Check sheet for the modelled part. Datum: model origin and axes. Units: mm. Face numbers are marked on the shaded views. A direction names the side the tool comes from. Give positions to 0.01 mm unless a question says otherwise; leave off trailing zeros. Loops run counter-clockwise (first coordinate to the right, second up) from the corner with the lowest first, then second, coordinate; pieces in that order, holes last. Notation, with made-up numbers: (41, 18.25) - (82, 18.25) arc R21 ccw to (82, 23.25) - close; hole circle Ø4 at (18.25, 0.25). An arc over 180 degrees is marked (long way). Use CSV: the item, a comma, the result in double quotes.
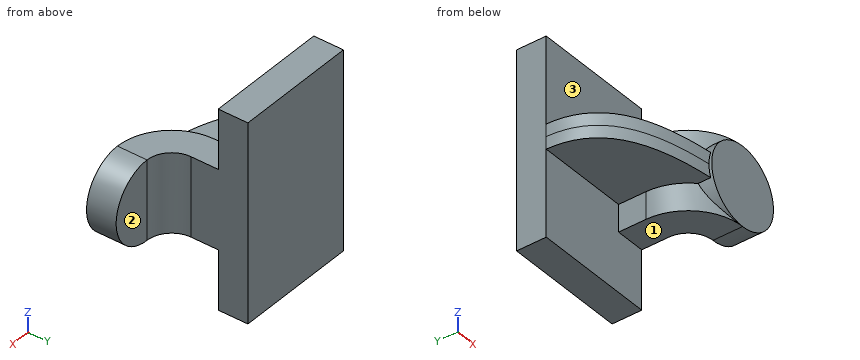
from build123d import *

# Parameters (mm, degrees)
F1_DEPTH = 63.5
F2_DEPTH = 25.4
F3_DEPTH = 7.9375
F0_W     = 25.4
F0_H     = 19.0500014678


with BuildPart() as f1:
    # F0 (on Top) → F1 (new body, symmetric)
    with BuildSketch(Plane.XY):
        Polygon((39.2749942839, 9.525), (-39.2749942839, 9.525), (-39.2749942839, -9.525), (20.2249928161, -9.525), (39.2749942839, -9.525), align=None)
    extrude(amount=F1_DEPTH, both=True)

    # F0 (on Top) → F2 (join, symmetric)
    with BuildSketch(Plane.XY):
        with BuildLine():
            Line((39.2749942839, -27.0002), (39.2749942839, -9.525))
            Line((39.2749942839, -9.525), (20.2249928161, -9.525))
            Line((20.2249928161, -9.525), (20.2249928161, -27.0002))
            ThreePointArc((20.2249928161, -27.0002), (29.3367398508, -50.5253274831), (51.9175683258, -61.7752938165))
            add(Edge.make_bspline(
                [(51.9175683258, -61.7752938165), (52.9952696281, -61.8278519925), (54.0729461799, -61.8776803226), (55.1499942839, -61.9252014678)],
                knots=[105.4761775762, 105.4761775762, 105.4761775762, 105.4761775762, 107.990090193, 107.990090193, 107.990090193, 107.990090193], degree=3))
            Line((55.1499942839, -61.9252014678), (55.1499942839, -42.8752))
            ThreePointArc((55.1499942839, -42.8752), (43.9246741326, -38.2255201513), (39.2749942839, -27.0002))
        make_face()
    extrude(amount=F2_DEPTH, both=True)

    # F0 (on Top) → F3 (join, symmetric)
    with BuildSketch(Plane.XY):
        with BuildLine():
            Line((20.2249928161, -9.525), (-39.2749942839, -9.525))
            add(Edge.make_bspline(
                [(-39.2749942839, -9.525), (-38.560182874, -52.5593411678), (6.7004779731, -59.5701115574), (51.9175683258, -61.7752938165)],
                knots=[0, 0, 0, 0, 105.4761775762, 105.4761775762, 105.4761775762, 105.4761775762], degree=3))
            ThreePointArc((51.9175683258, -61.7752938165), (29.3367398508, -50.5253274831), (20.2249928161, -27.0002))
            Line((20.2249928161, -27.0002), (20.2249928161, -9.525))
        make_face()
    extrude(amount=F3_DEPTH, both=True)

    # F0 (on Top) → F4 (revolve)
    with BuildSketch(Plane.XY):
        with Locations((67.8499942839, -52.4002007339)):
            Rectangle(F0_W, F0_H)
    revolve(axis=Axis((55.1499942839, -52.3875, 0), (0, -1, 0)))


solid = f1.part
1. Sectioned sample at D-D, the plane z = -45.5. Record the boundary of the cut face in (x, y) (3 decimals).
Completed:
outline,"(-39.275, -9.525) - (39.275, -9.525) - (39.275, 9.525) - (-39.275, 9.525) - close"
2. Go/stop test with flat-tipped pins: pin 1 Ø8.5 at (y, z) = (-15.5, 14.5) entering from -X (3 decimals); pin 2 Ø2 at (y, z) = (-19, -2.5) entering from -X; pin 3 Ø2 at (x, z) = (34, 23) entering from -Y. Record where each tip stops, or that it passes through.
Completed:
pin 1,"stops at x = 20.225"
pin 2,"stops at x = -38.49"
pin 3,"stops at y = -55.53"
3. Set-up check for the marked faces 1, 2 and 3: record each of +Z, -Z, +X, -X, +Y, -Y from which the full face is reachable in a straight line by a thin tool's end or side.
Completed:
face 1,"-Z, +X, -X, -Y"
face 2,"+Z, -Z, +X, +Y"
face 3,"+Z, -X, -Y"
4. Sectioned sample at C-C, the plane z = -14. Record the boundary of the cut face in (x, y) (3 decimals), and give its area (3 significant figures).
Completed:
outline,"(-39.275, -9.525) - (20.225, -9.525) - (20.225, -27) arc R34.925 ccw to (33.957, -54.76) - (33.957, -61.925) - (76.343, -61.925) - (76.343, -42.875) - (55.15, -42.875) arc R15.875 cw to (39.275, -27) - (39.275, 9.525) - (-39.275, 9.525) - close"
area,"3,040 mm²"
5. Sectioned sample at B-B, the plane x = 63.5. Record the boundary of the cut face in (y, z), and give its area (3 significant figures).
Completed:
outline,"(-61.93, -23.99) - (-42.88, -23.99) - (-42.88, 23.99) - (-61.93, 23.99) - close"
area,"914 mm²"
6. Scan lines: line 1 along X through (y, z) = (-5.5, -28) (3 decimals); line 2 along Z through (x, y) = (-11, -32); line 3 along Y through (x, z) = (65, -18). Record each from-to range of solid material in increasing order.
Completed:
line 1,"x = -39.275 to 39.275"
line 2,"z = -7.94 to 7.94"
line 3,"y = -61.93 to -42.88"
7. Sectioned sample at A-A, the plane z = 19.5. Record the boundary of the cut face in (x, y) (3 decimals), and give its area (3 significant figures).
Completed:
outline,"(-39.275, -9.525) - (20.225, -9.525) - (20.225, -27) arc R34.925 ccw to (38.874, -57.901) - (38.874, -61.925) - (71.426, -61.925) - (71.426, -42.875) - (55.15, -42.875) arc R15.875 cw to (39.275, -27) - (39.275, 9.525) - (-39.275, 9.525) - close"
area,"2,920 mm²"
